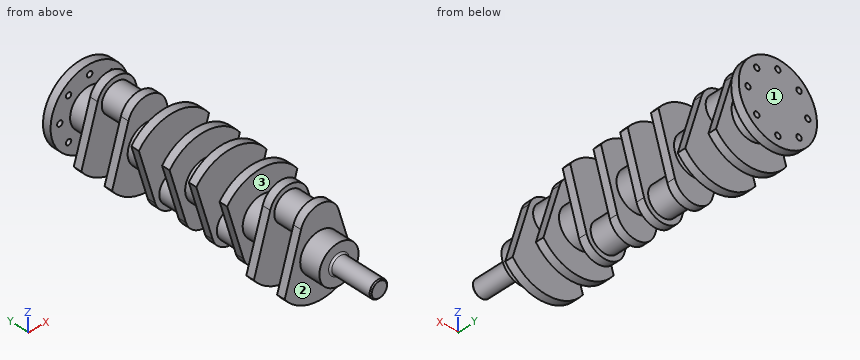
from build123d import *

# Parameters (mm, degrees)
SKETCH1_R              = 16
BOSS_EXTRUDE1_DEPTH    = 80
BOSS_EXTRUDE2_START    = 80
SKETCH1_3_R            = 36
SKETCH1_3_R_2          = 16
BOSS_EXTRUDE2_DEPTH    = 38
BOSS_EXTRUDE3_DEPTH    = 15
SKETCH2_3_R            = 27
BOSS_EXTRUDE4_DEPTH    = 61
LPATTERN1_COUNT        = 2
LPATTERN1_PITCH        = 61
SKETCH3_R              = 36
BOSS_EXTRUDE5_DEPTH    = 38
BOSS_EXTRUDE6_START    = 38
BOSS_EXTRUDE6_DEPTH    = 15
SKETCH6_R              = 27
BOSS_EXTRUDE8_DEPTH    = 46
LPATTERN3_COUNT        = 2
LPATTERN3_PITCH        = 61
LPATTERN5_COUNT        = 2
LPATTERN5_PITCH        = 114
LPATTERN5_START        = 38
LPATTERN5_COPY_1_DEPTH = 15
LPATTERN6_COUNT        = 2
LPATTERN6_PITCH        = 342
LPATTERN6_COPY_1_DEPTH = 15
SKETCH7_R              = 36
BOSS_EXTRUDE9_DEPTH    = 38
SKETCH8_R              = 72
SKETCH8_R_2            = 5
BOSS_EXTRUDE10_DEPTH   = 15
CHAMFER1_SIZE          = 2
FILLET1_R              = 3


with BuildPart() as part:
    # Sketch1 → Boss-Extrude1 (new body)
    with BuildSketch(Plane(origin=(0, 0, 0), x_dir=(1, 0, 0), z_dir=(0, 1, 0))):
        with Locations(Location((0, 0, 0), (0, 0, 270))):
            Circle(SKETCH1_R)
    extrude(amount=BOSS_EXTRUDE1_DEPTH)

    # Sketch1<3> → Boss-Extrude2 (add)
    # profile 1 of 2: a face of its own
    with BuildSketch(Plane(origin=(0, 0, 0), x_dir=(1, 0, 0), z_dir=(0, 1, 0)).offset(BOSS_EXTRUDE2_START)):
        with Locations(Location((0, 0, 0), (0, 0, 270))):
            Circle(SKETCH1_3_R)
        with Locations(Location((0, 0, 0), (0, 0, 270))):
            Circle(SKETCH1_3_R_2, mode=Mode.SUBTRACT)
    # profile 2 of 2: a face of its own
    with BuildSketch(Plane(origin=(0, 0, 0), x_dir=(1, 0, 0), z_dir=(0, 1, 0)).offset(BOSS_EXTRUDE2_START)):
        with Locations(Location((0, 0, 0), (0, 0, 270))):
            Circle(SKETCH1_3_R_2)
    boss_extrude2 = extrude(amount=BOSS_EXTRUDE2_DEPTH)

    # Sketch2 → Boss-Extrude3 (add)
    with BuildSketch(Plane(origin=(0, 118, 0), x_dir=(1, 0, 0), z_dir=(0, 1, 0))):
        with BuildLine():
            Line((-34.517510455, -54.224552409), (-64.569893475, 47.23059238))
            ThreePointArc((-64.569893475, 47.23059238), (0, 80), (64.569893475, 47.23059238))
            Line((64.569893475, 47.23059238), (34.517510455, -54.224552409))
            ThreePointArc((34.517510455, -54.224552409), (0, -80), (-34.517510455, -54.224552409))
        make_face()
    boss_extrude3 = extrude(amount=BOSS_EXTRUDE3_DEPTH)

    # Sketch2<3> → Boss-Extrude4 (add)
    with BuildSketch(Plane(origin=(0, 118, 0), x_dir=(1, 0, 0), z_dir=(0, 1, 0))):
        with Locations(Location((0, -44, 0), (0, 0, 90))):
            Circle(SKETCH2_3_R)
    boss_extrude4 = extrude(amount=BOSS_EXTRUDE4_DEPTH)

    # LPattern1: Boss-Extrude3 ×2
    with Locations(*[(0, i * LPATTERN1_PITCH, 0) for i in range(1, LPATTERN1_COUNT)]):
        add(boss_extrude3)

    # Sketch3 → Boss-Extrude5 (add)
    with BuildSketch(Plane(origin=(0, 194, 0), x_dir=(1, 0, 0), z_dir=(0, 1, 0))):
        with Locations(Location((0, 0, 0), (0, 0, 270))):
            Circle(SKETCH3_R)
    boss_extrude5 = extrude(amount=BOSS_EXTRUDE5_DEPTH)

    # Sketch5 → Boss-Extrude6 (add)
    with BuildSketch(Plane(origin=(0, 194, 0), x_dir=(1, 0, 0), z_dir=(0, 1, 0)).offset(BOSS_EXTRUDE6_START)):
        with BuildLine():
            Line((-34.517510455, 54.224552409), (-64.569893475, -47.23059238))
            ThreePointArc((-64.569893475, -47.23059238), (0, -80), (64.569893475, -47.23059238))
            Line((64.569893475, -47.23059238), (34.517510455, 54.224552409))
            ThreePointArc((34.517510455, 54.224552409), (0, 80), (-34.517510455, 54.224552409))
        make_face()
    boss_extrude6 = extrude(amount=BOSS_EXTRUDE6_DEPTH)

    # Sketch6 → Boss-Extrude8 (add)
    with BuildSketch(Plane(origin=(0, 247, 0), x_dir=(1, 0, 0), z_dir=(0, 1, 0))):
        with Locations(Location((0, 44, 0), (0, 0, 90))):
            Circle(SKETCH6_R)
    boss_extrude8 = extrude(amount=BOSS_EXTRUDE8_DEPTH)

    # LPattern3: Boss-Extrude6 ×2
    with Locations(*[(0, i * LPATTERN3_PITCH, 0) for i in range(1, LPATTERN3_COUNT)]):
        add(boss_extrude6)

    # LPattern5: Boss-Extrude5, Boss-Extrude6, Boss-Extrude8 ×2
    with Locations(*[(0, i * LPATTERN5_PITCH, 0) for i in range(1, LPATTERN5_COUNT)]):
        add(boss_extrude5)
        add(boss_extrude6)
        add(boss_extrude8)

    # LPattern5 copy 1 sketch → LPattern5 copy 1 (add)
    with BuildSketch(Plane(origin=(0, 369, 0), x_dir=(1, 0, 0), z_dir=(0, 1, 0)).offset(LPATTERN5_START)):
        with BuildLine():
            Line((-34.517510455, 54.224552409), (-64.569893475, -47.23059238))
            ThreePointArc((-64.569893475, -47.23059238), (0, -80), (64.569893475, -47.23059238))
            Line((64.569893475, -47.23059238), (34.517510455, 54.224552409))
            ThreePointArc((34.517510455, 54.224552409), (0, 80), (-34.517510455, 54.224552409))
        make_face()
    extrude(amount=LPATTERN5_COPY_1_DEPTH)

    # LPattern6: Boss-Extrude2, Boss-Extrude3, Boss-Extrude4 ×2
    with Locations(*[(0, i * LPATTERN6_PITCH, 0) for i in range(1, LPATTERN6_COUNT)]):
        add(boss_extrude2)
        add(boss_extrude3)
        add(boss_extrude4)

    # LPattern6 copy 1 sketch → LPattern6 copy 1 (add)
    with BuildSketch(Plane(origin=(0, 521, 0), x_dir=(1, 0, 0), z_dir=(0, 1, 0))):
        with BuildLine():
            Line((-34.517510455, -54.224552409), (-64.569893475, 47.23059238))
            ThreePointArc((-64.569893475, 47.23059238), (0, 80), (64.569893475, 47.23059238))
            Line((64.569893475, 47.23059238), (34.517510455, -54.224552409))
            ThreePointArc((34.517510455, -54.224552409), (0, -80), (-34.517510455, -54.224552409))
        make_face()
    extrude(amount=LPATTERN6_COPY_1_DEPTH)

    # Sketch7 → Boss-Extrude9 (add)
    with BuildSketch(Plane(origin=(0, 536, 0), x_dir=(1, 0, 0), z_dir=(0, 1, 0))):
        with Locations(Location((0, 0, 0), (0, 0, 270))):
            Circle(SKETCH7_R)
    extrude(amount=BOSS_EXTRUDE9_DEPTH)

    # Sketch8 → Boss-Extrude10 (add)
    with BuildSketch(Plane(origin=(0, 574, 0), x_dir=(1, 0, 0), z_dir=(0, 1, 0))):
        with Locations(Location((0, 0, 0), (0, 0, 270))):
            Circle(SKETCH8_R)
        with Locations(Location((0, 55, 0), (0, 0, 270))):
            Circle(SKETCH8_R_2, mode=Mode.SUBTRACT)
        with Locations(Location((38.890872965, 38.890872965, 0), (0, 0, 270))):
            Circle(SKETCH8_R_2, mode=Mode.SUBTRACT)
        with Locations(Location((55, 0, 0), (0, 0, 270))):
            Circle(SKETCH8_R_2, mode=Mode.SUBTRACT)
        with Locations(Location((38.890872965, -38.890872965, 0), (0, 0, 270))):
            Circle(SKETCH8_R_2, mode=Mode.SUBTRACT)
        with Locations(Location((0, -55, 0), (0, 0, 270))):
            Circle(SKETCH8_R_2, mode=Mode.SUBTRACT)
        with Locations(Location((-38.890872965, -38.890872965, 0), (0, 0, 270))):
            Circle(SKETCH8_R_2, mode=Mode.SUBTRACT)
        with Locations(Location((-55, 0, 0), (0, 0, 270))):
            Circle(SKETCH8_R_2, mode=Mode.SUBTRACT)
        with Locations(Location((-38.890872965, 38.890872965, 0), (0, 0, 270))):
            Circle(SKETCH8_R_2, mode=Mode.SUBTRACT)
    extrude(amount=BOSS_EXTRUDE10_DEPTH)

    # Chamfer1
    chamfer1_edges = [part.edges().sort_by_distance(p)[0] for p in [
        (0, 0, -16),
    ]]
    chamfer(chamfer1_edges, length=CHAMFER1_SIZE)

    # Fillet1
    fillet1_edges = [part.edges().sort_by_distance(p)[0] for p in [
        (0, 80, -16),
    ]]
    fillet(fillet1_edges, radius=FILLET1_R)


solid = part.part
Design review of the part built by this model. Coordinates are the model's own, in mm. Face numbers are marked on the shaded views. Coordinates: 2 decimals unless noted, no trailing zeros. Loops run counter-clockwise (first coordinate to the right, second up) from the corner with the lowest first, then second, coordinate; pieces in that order, holes last.
Item 1: Wall thickness on L1, parallel to Y at x = -12.5, z = -22; L2, parallel to Y at x = 3, z = -58; L3, parallel to Y at x = -13, z = -16: over which ranges is each line inside the solid? List them lowest first.
Completed:
L1: y = 80 to 133, 179 to 475, 521 to 589
L2: y = 118 to 133, 179 to 194, 232 to 308, 346 to 422, 460 to 475, 521 to 536
L3: y = 80 to 133, 179 to 247, 293 to 361, 407 to 475, 521 to 589
Item 2: Add section A-A (y = 353.5). Write out the cut boundary in (x, z).
Completed:
outline: (-64.57, 47.23) - (-34.52, -54.22) arc R36 ccw to (34.52, -54.22) - (64.57, 47.23) arc R80 ccw to start
Item 3: Add section B-B (y = 511.5). Write out the cut boundary in (x, z).
Completed:
outline: circle Ø54 at (0, 44)
Item 4: Clearance check with flat-ended pins moving along their axes: pin 1 (16 mm diameter, centred on x = 0, z = -55, fed in from +Y); pin 2 (1 mm diameter, centred on x = -38.5, z = -6, fed in from -Y); pin 3 (1.5 mm diameter, centred on y = 334.5, z = 38.5, fed in from +X); pin 4 (6 mm diameter, centred on x = 7, y = 88, fed in from +Z). State where each tip first meets the part, or that it passes through.
Completed:
pin 1: stops at y = 589
pin 2: stops at y = 118
pin 3: passes through
pin 4: stops at z = 35.78
Item 5: Draft analysis for pull direction Y (two halves, no side actions). For the marked faces 1, 2 and 3, state which applies: pulls with the +Y half, pulls with the -Y half, needs draft (parallel to the pull), parting line crosses it, or undercut.
Completed:
face 1: pulls with the +Y half
face 2: pulls with the -Y half
face 3: undercut
